Can you work these out from the drawing? Everything is in mm from the part's minimum corner. Coordinates: 2 decimals unless noted, no trailing zeros. Order: outer loops, then holes, each group sorted by start corner. A loop starts at its lowest first (then second) coordinate and runs counter-clockwise, first axis right, second up. Notation, with made-up numbers: M 25.25,1 L 72.25,1 A20 cw 72.25,35 Z; hole C -10.5,-4 d3. An arc over 180 degrees is marked long. One line per question, with ' | ' between items. Start each with the question number.
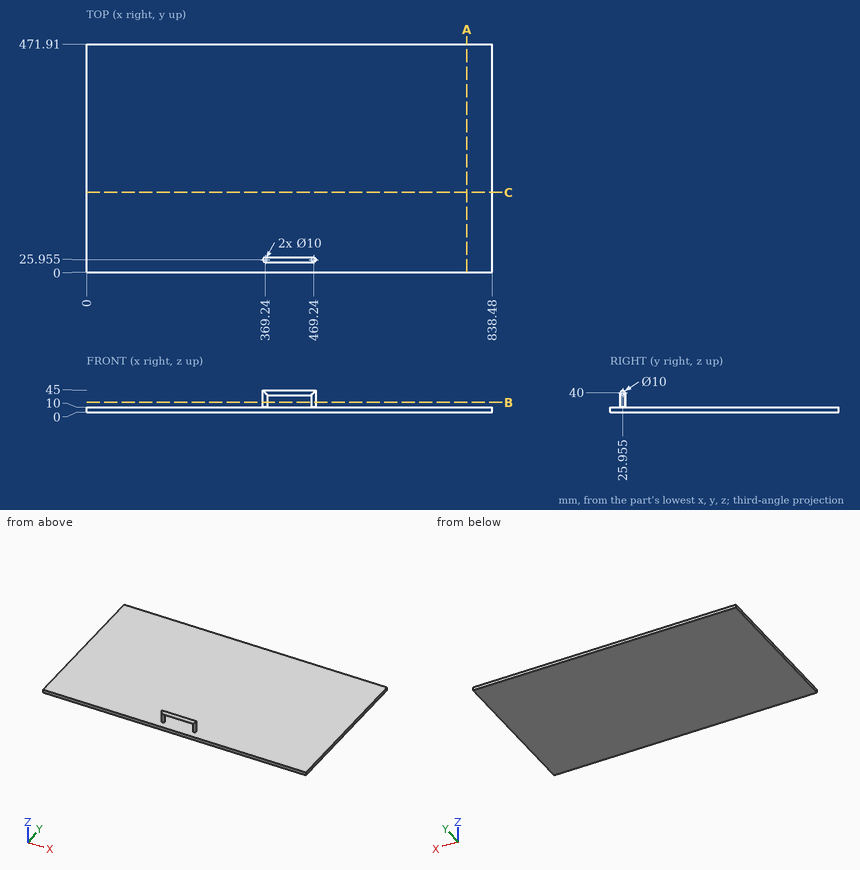
(1) Imagine slicing it at C-C, the plane y = 165. Write out the boundary of the cut face in (x, z), plus the area to 3 significant figures.
(2) Imagine slicing it at B-B, the plane z = 20. Write out the boundary of the cut face in (x, y) (3 decimals), plus the area to 3 significant figures.
(3) Imagine slicing it at A-A, the plane x = 786. Write out the boundary of the cut face in (y, z).
(4) If I drill on line 1 along Z through (x, y) = (590, 324.5), over which ranges is the centre line in solid material (lowest first)? Write a range as from..to.
(5) For P1, Ø5, axis at x = 98, y = 51.5, coming from the -Z side; P2, Ø12, axis at x = 463.5, z = 22, coming from the -Y side (3 decimals); P3, Ø3, axis at x = 234, y = 351.5, coming from the +Z side, each with a flat end and sliding along its axis, tell me the tip position at first contact or that it passes through.
Answers:
1) outline: M 0,0 L 838.48,0 L 838.48,10 L 0,10 Z | area: 8,380 mm²
2) outline: C 369.24,25.955 d10; C 469.24,25.955 d10 | area: 157 mm²
3) outline: M 0,0 L 471.91,0 L 471.91,10 L 0,10 Z
4) line 1: 0..10
5) P1: z = 0 | P2: y = 20.955 | P3: z = 10
